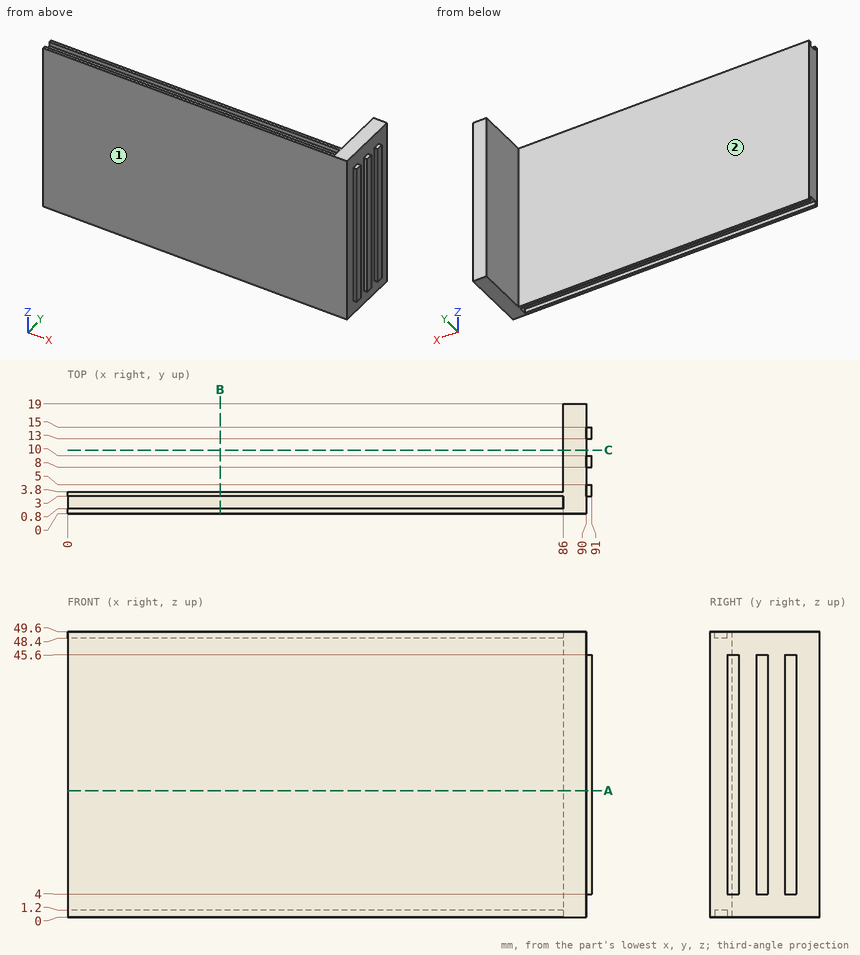
Check sheet for the drawn part. Datum: minimum x, y, z corner. Units: mm. A direction names the side the tool comes from. Round coordinates to 2 decimals unless told otherwise and drop trailing zeros. Loops run counter-clockwise (first coordinate to the right, second up) from the corner with the lowest first, then second, coordinate; pieces in that order, holes last. Notation, with made-up numbers: (-12.75, -14) -> (-2.75, -14) arc R17 ccw to (-2.75, -1) -> close; hole circle Ø7 at (-36, -20). An arc over 180 degrees is marked (long way). Put each result on its own line as item: value. Start each with the question number.
1. Scan lines: probe 1 along X at (y, z) = (10.25, 22); probe 2 along Y at (x, z) = (16, 20.5); probe 3 along X at (y, z) = (14.25, 17.5). Record each from-to range of solid material in increasing order.
2. Gauge pin test, flat ends, axial feed: pin 1 (0.8 mm diameter, centred on x = 90.5, z = 31.5, fed in from +Y); pin 2 (8 mm diameter, centred on x = 55, z = 38.5, fed in from +Y); pin 3 (1.1 mm diameter, centred on x = 52.5, y = 1.5, fed in from +Z). Record the tip position at first contact, or that the pin passes through.
3. Access from +Z, -Z, +X, -X, +Y, -Y to the whole of each face (thin tool, end or side, straight path). Record for the marked faces 1 and 2.
4. Section check C-C (y = 11). Enter the section's corners in (x, z), plus the area to 3 significant figures.
5. Section check B-B (x = 26.5). Enter the section's corners in (y, z).
6. Section check A-A (z = 22). Enter the section's corners in (x, y), plus the area to 3 significant figures.
Findings:
1. probe 1: x = 86 to 90
1. probe 2: y = 0 to 3.8
1. probe 3: x = 86 to 91
2. pin 1: stops at y = 15
2. pin 2: stops at y = 3.8
2. pin 3: stops at z = 48.4
3. face 1: +Z, -Z, +X, -X, -Y
3. face 2: +Z, -Z, -X, +Y
4. outline: (86, 0) -> (90, 0) -> (90, 49.6) -> (86, 49.6) -> close
4. area: 198 mm^2
5. outline: (0, 0) -> (0.8, 0) -> (0.8, 1.2) -> (3, 1.2) -> (3, 0) -> (3.8, 0) -> (3.8, 49.6) -> (3, 49.6) -> (3, 48.4) -> (0.8, 48.4) -> (0.8, 49.6) -> (0, 49.6) -> close
6. outline: (0, 0) -> (90, 0) -> (90, 3) -> (91, 3) -> (91, 5) -> (90, 5) -> (90, 8) -> (91, 8) -> (91, 10) -> (90, 10) -> (90, 13) -> (91, 13) -> (91, 15) -> (90, 15) -> (90, 19) -> (86, 19) -> (86, 3.8) -> (0, 3.8) -> close
6. area: 409 mm^2
